from build123d import *

# Parameters (mm, degrees)
F0_W     = 45.212
F0_H     = 46.99
F1_DEPTH = 1.5875
F2_W     = 30.48
F2_H     = 30.48
F3_DEPTH = 6.35
F4_R     = 2.921
F4_R_2   = 1.016
F5_DEPTH = 10.16
F6_DEPTH = 6.35


with BuildPart() as f1:
    # F0 (on Top) → F1 (new body)
    with BuildSketch(Plane.XY):
        Rectangle(F0_W, F0_H)
    extrude(amount=F1_DEPTH)

    # F2 (on face) → F3 (cut)
    with BuildSketch(Plane.XY.offset(1.5875)):
        Rectangle(F2_W, F2_H)
    extrude(amount=-F3_DEPTH, mode=Mode.SUBTRACT)

    # F4 (on face) → F5 (join)
    with BuildSketch(Plane.XY.offset(1.5875)):
        with Locations((19.6215, -20.5105)):
            Circle(F4_R)
        with Locations((19.6215, -20.5105)):
            Circle(F4_R_2, mode=Mode.SUBTRACT)
        with BuildLine():
            ThreePointArc((-22.606, 19.9047486071), (-19.4439646983, 17.6054183746), (-16.8275, 20.5105))
            ThreePointArc((-16.8275, 20.5105), (-19.4439646983, 23.4155816254), (-22.606, 21.1162513929))
            Line((-22.606, 21.1162513929), (-22.606, 19.9047486071))
        make_face()
        with BuildLine():
            ThreePointArc((-16.8275, -20.5105), (-19.4439646983, -17.6054183746), (-22.606, -19.9047486071))
            Line((-22.606, -19.9047486071), (-22.606, -21.1162513929))
            ThreePointArc((-22.606, -21.1162513929), (-19.4439646983, -23.4155816254), (-16.8275, -20.5105))
        make_face()
        with Locations((19.6215, 20.5105)):
            Circle(F4_R)
        with Locations((19.6215, 20.5105)):
            Circle(F4_R_2, mode=Mode.SUBTRACT)
    extrude(amount=F5_DEPTH)

    # F4 (on face) → F6 (cut)
    with BuildSketch(Plane.XY.offset(1.5875)):
        with Locations((19.6215, -20.5105)):
            Circle(F4_R_2)
        with Locations((19.6215, 20.5105)):
            Circle(F4_R_2)
    extrude(amount=-F6_DEPTH, mode=Mode.SUBTRACT)


solid = f1.part
Can you work these out from the model? Positions are in its coordinate system, mm. A direction names the side the tool comes from. Coordinates: 2 decimals unless noted, no trailing zeros. Write each loop counter-clockwise with the first axis right and the second up, starting at its lowest first coordinate (ties: lowest second). Pieces come first, ordered by that corner, then holes. Notation, with made-up numbers: (-28, 3) - (29, 3) arc R22 ccw to (29, 9) - close; hole circle Ø9 at (10.5, -29). An arc over 180 degrees is marked (long way). Return JSON: item names as keys, results as strings. Group by question number.
Item 1: If we section it at D-D (z = 1): Write out the boundary of the cut face in (x, y) (1 decimal).
Item 2: I'm going to push a flat-ended pin straight in: pin 1 Ø4 at (x, z) = (5, 4.5) entering from -Y. Where does the tip first touch, or does it pass through?
Item 3: Which directions (+Z, -Z, +X, -X, +Y, -Y) give clear straight access to the entire face, cutting with the end or side of a thin tool? Please do faces 5 (the face through (19.241, -17.614, 6.596)), 6 (the face through (-20, 21, 11.748)), 7 (the face through (0, -15.24, 1)).
Item 4: If we section it at A-A (y = 10.5): Write out the boundary of the cut face in (x, z), then the cut area to 3 significant figures.
Item 5: If we section it at C-C (x = 13.5): Write out the boundary of the cut face in (y, z) (1 decimal).
Item 6: Please list where these lines run through material, in increasing order: probe 1 along X at (y, z) = (-10, 0.75); probe 2 along Z at (x, y) = (-9.5, 20.5); probe 3 along X at (y, z) = (18.5, 3.75).
Item 7: We'd pull the mould along X, two halves only. Please class faces 1 (the face through (-15.4, 0.3, 0)), 2 (the face through (-22.606, 0, 1)), 3 (the face through (22.606, 0, 1)), 4 (the face through (15.24, 0, 1)): pulls with the +X half, pulls with the -X half, needs draft (parallel to the pull), parting line crosses it, or undercut.
Item 8: If we section it at B-B (z = 5.75): Write out the boundary of the cut face in (x, y), then the cut area to 3 significant figures.
Return value:
{
 "1": {"outline": "(-22.6, -23.5) - (22.6, -23.5) - (22.6, 23.5) - (-22.6, 23.5) - close; hole (-15.2, -15.2) - (15.2, -15.2) - (15.2, 15.2) - (-15.2, 15.2) - close; hole circle Ø2 at (19.6, -20.5); hole circle Ø2 at (19.6, 20.5)"},
 "2": {"pin 1": "passes through"},
 "3": {"face 5": "+Z", "face 6": "+Z, +X, -X, +Y, -Y", "face 7": "+Z, -Z"},
 "4": {"outline": "(-22.61, 0) - (-15.24, 0) - (-15.24, 1.59) - (-22.61, 1.59) - close; (15.24, 0) - (22.61, 0) - (22.61, 1.59) - (15.24, 1.59) - close", "area": "23.4 mm^2"},
 "5": {"outline": "(-23.5, 0) - (-15.2, 0) - (-15.2, 1.6) - (-23.5, 1.6) - close; (15.2, 0) - (23.5, 0) - (23.5, 1.6) - (15.2, 1.6) - close"},
 "6": {"probe 1": "x = -22.61 to -15.24, 15.24 to 22.61", "probe 2": "z = 0 to 1.59", "probe 3": "x = -21.87 to -17.63, 17.5 to 21.74"},
 "7": {"face 1": "needs draft", "face 2": "pulls with the -X half", "face 3": "pulls with the +X half", "face 4": "undercut"},
 "8": {"outline": "(-22.61, -21.12) arc R2.92 ccw (long way) to (-22.61, -19.9) - close; (-22.61, 19.9) arc R2.92 ccw (long way) to (-22.61, 21.12) - close; circle Ø5.84 at (19.62, -20.51); circle Ø5.84 at (19.62, 20.51); hole circle Ø2.03 at (19.62, -20.51); hole circle Ø2.03 at (19.62, 20.51)", "area": "101 mm^2"}
}
